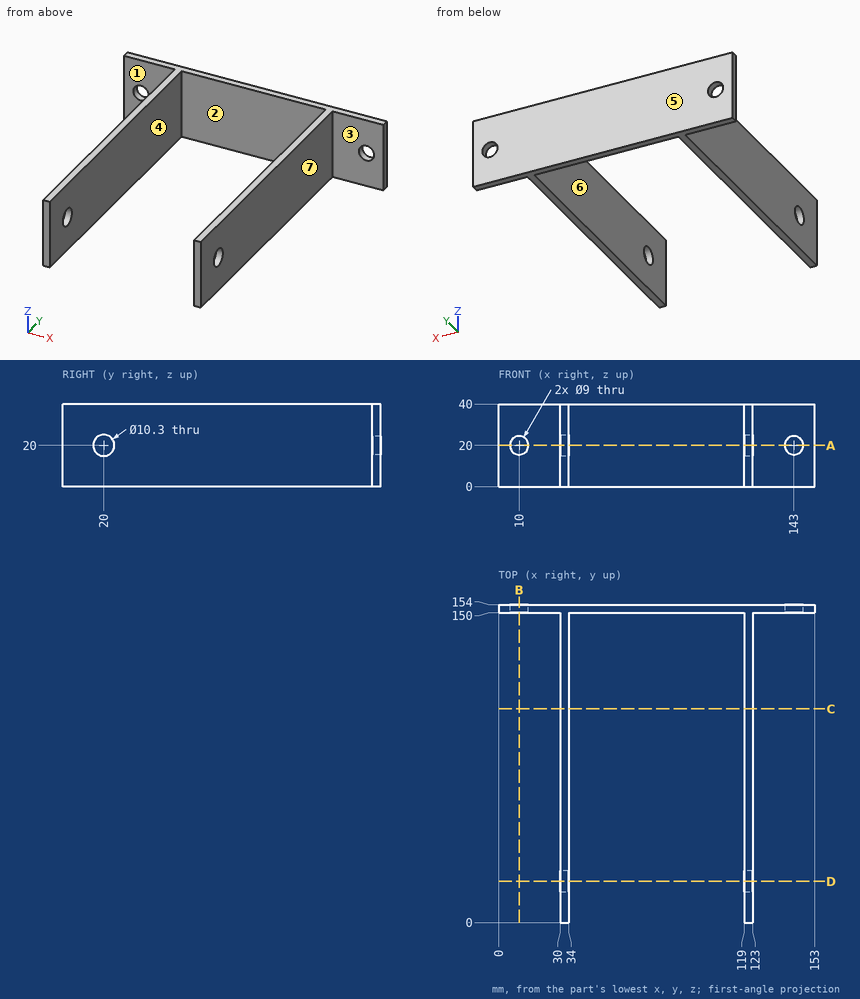
Study the drawing (mm; zero at the part's minimum x, y, z) and answer. A direction names the side the tool comes from. Give positions to 0.01 mm unless a question says otherwise; leave off trailing zeros. Loops run counter-clockwise (first coordinate to the right, second up) from the corner with the lowest first, then second, coordinate; pieces in that order, holes last. Notation, with made-up numbers: (68.5, 60) - (95.5, 60) arc R30 ccw to (95.5, 96) - close; hole circle Ø11 at (48.25, 2). An arc over 180 degrees is marked (long way). Return JSON: item names as keys, results as strings. Group by question number.
1. Determine the mould class of the marked faces 4, 5, 6 and 7 for opening direction X: pulls with the +X half, pulls with the -X half, needs draft (parallel to the pull), parting line crosses it, or undercut.
2. Straight lines are drawn through the part: line 1 (X direction, y = 100, z = 27); line 2 (Z direction, x = 10, y = 150.9); line 3 (Z direction, x = 31, y = 20). For each, find the intervals that lie inside material, in ascending order. Write a range as [from, to].
3. Which of the six approach directions +Z, -Z, +X, -X, +Y, -Y give full straight-line access (tool end or side, diameter ignored) to the marked faces 1, 2 and 3?
4. Given pin 1 Ø8 at (x, z) = (10, 20) entering from +Y; pin 2 Ø8 at (y, z) = (122.5, 10.5) entering from -X; pin 3 Ø1.5 at (y, z) = (111.5, 5.5) entering from +X; pin 4 Ø9 at (x, z) = (18, 15.5) entering from -Y, each flat-ended and moving along its own axis, determine where each tip first touches the part or whether it passes through.
5. Find section C-C (y = 103.5). Write down the section's boundary in (x, z).
6. Find section B-B (x = 10). Write down the section's boundary in (y, z), then the cut area to 3 significant figures.
7. Find section D-D (y = 20). Write down the section's boundary in (x, z), then the cut area to 3 significant figures.
8. Find section A-A (z = 20). Write down the section's boundary in (x, y), then the cut area to 3 significant figures.
Verdict:
{
 "1": {"face 4": "undercut", "face 5": "needs draft", "face 6": "undercut", "face 7": "pulls with the +X half"},
 "2": {"line 1": "x = [30, 34], [119, 123]", "line 2": "z = [0, 15.5], [24.5, 40]", "line 3": "z = [0, 14.85], [25.15, 40]"},
 "3": {"face 1": "+Z, -Z, -X, -Y", "face 2": "+Z, -Z, -Y", "face 3": "+Z, -Z, +X, -Y"},
 "4": {"pin 1": "passes through", "pin 2": "stops at x = 30", "pin 3": "stops at x = 123", "pin 4": "stops at y = 150"},
 "5": {"outline": "(30, 0) - (34, 0) - (34, 40) - (30, 40) - close; (119, 0) - (123, 0) - (123, 40) - (119, 40) - close"},
 "6": {"outline": "(150, 0) - (154, 0) - (154, 15.5) - (150, 15.5) - close; (150, 24.5) - (154, 24.5) - (154, 40) - (150, 40) - close", "area": "124 mm^2"},
 "7": {"outline": "(30, 0) - (34, 0) - (34, 14.85) - (30, 14.85) - close; (30, 25.15) - (34, 25.15) - (34, 40) - (30, 40) - close; (119, 0) - (123, 0) - (123, 14.85) - (119, 14.85) - close; (119, 25.15) - (123, 25.15) - (123, 40) - (119, 40) - close", "area": "238 mm^2"},
 "8": {"outline": "(0, 150) - (5.5, 150) - (5.5, 154) - (0, 154) - close; (14.5, 150) - (30, 150) - (30, 25.15) - (34, 25.15) - (34, 150) - (119, 150) - (119, 25.15) - (123, 25.15) - (123, 150) - (138.5, 150) - (138.5, 154) - (14.5, 154) - close; (30, 0) - (34, 0) - (34, 14.85) - (30, 14.85) - close; (119, 0) - (123, 0) - (123, 14.85) - (119, 14.85) - close; (147.5, 150) - (153, 150) - (153, 154) - (147.5, 154) - close", "area": "1,660 mm^2"}
}
